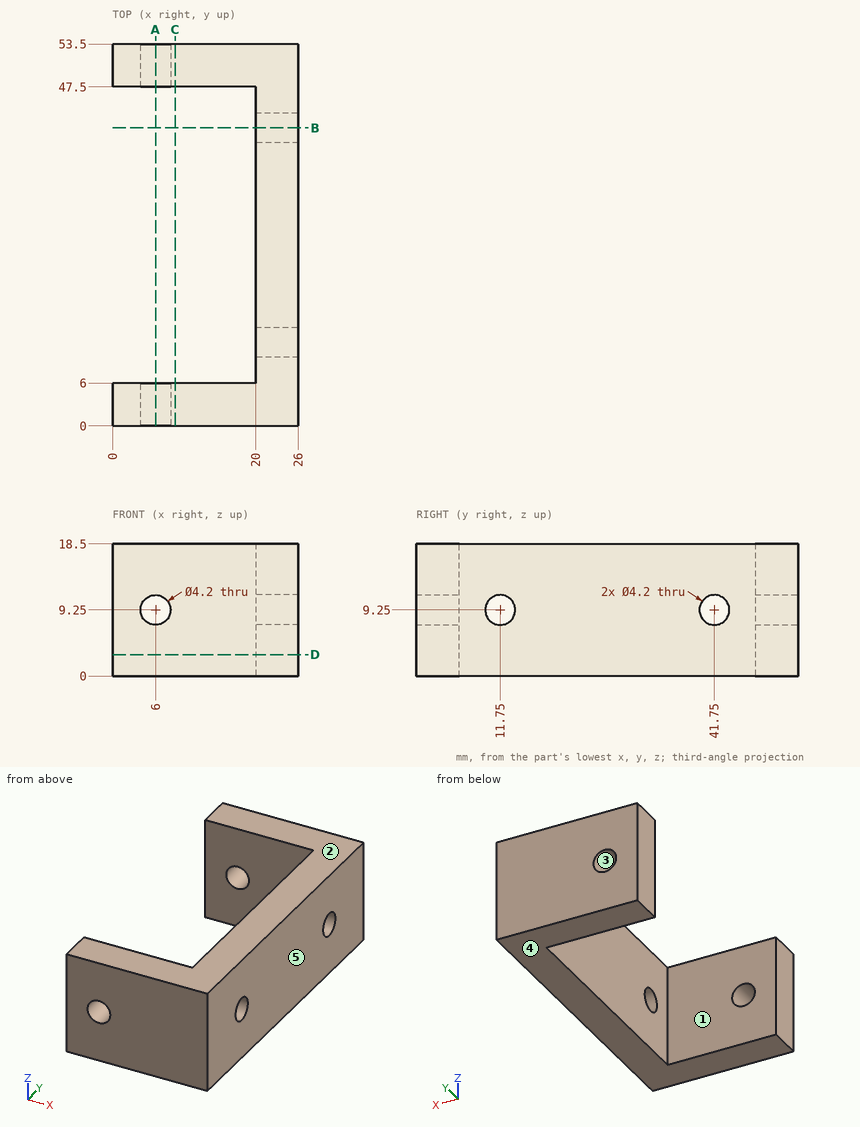
Design review of the part shown in the three views and the two pictorial views. Dimensions are in mm from the part's minimum x, y and z. A direction names the side the tool comes from. Round coordinates to 2 decimals unless told otherwise and drop trailing zeros. Write each loop counter-clockwise with the first axis right and the second up, starting at its lowest first coordinate (ties: lowest second). Pieces come first, ordered by that corner, then holes. Notation, with made-up numbers: (42.5, 43) -> (50.5, 43) arc R26 cw to (50.5, 78) -> close; hole circle Ø11 at (29, -20). An arc over 180 degrees is marked (long way). One line per question, with ' | ' between items. Start each with the question number.
1) Machinability: for the marked faces 1 and 2, which of the approach directions +Z, -Z, +X, -X, +Y, -Y give a long, thin tool a straight path to every point of the face, cutting with its end or side? Answer none if there is none.
2) Mouldability with a two-part tool opening along X and no side actions: class the marked faces 3, 4 and 5 as +X half, -X half, draft (parallel to the pull), parting line (faces both ways), or undercut.
3) Add section A-A (x = 6). Write out the cut boundary in (y, z).
4) Add section D-D (z = 3). Write out the cut boundary in (x, y).
5) Add section C-C (x = 8.75). Write out the cut boundary in (y, z), and give its area (3 significant figures).
6) Wall thickness on line 1 along Y through (x, z) = (10.5, 16); line 2 along Z through (x, y) = (6, 3.9); line 3 along X through (y, z) = (48.7, 9.25): over which ranges is each line inside the solid? List them lowest first.
7) For pin 1 Ø6.5 at (x, z) = (6, 9.25) entering from -Y; pin 2 Ø2.5 at (x, z) = (6, 9.25) entering from -Y; pin 3 Ø8 at (y, z) = (36, 2.5) entering from -X, all flat-tipped, find the tip position at first contact; note any pin that passes through.
8) Add section B-B (y = 41.75). Write out the cut boundary in (x, z), and give its area (3 significant figures).
Reported:
1) face 1: +Z, -Z, -X | face 2: +Z, +X, -X, +Y, -Y
2) face 3: undercut | face 4: draft | face 5: +X half
3) outline: (0, 0) -> (6, 0) -> (6, 7.15) -> (0, 7.15) -> close; (0, 11.35) -> (6, 11.35) -> (6, 18.5) -> (0, 18.5) -> close; (47.5, 0) -> (53.5, 0) -> (53.5, 7.15) -> (47.5, 7.15) -> close; (47.5, 11.35) -> (53.5, 11.35) -> (53.5, 18.5) -> (47.5, 18.5) -> close
4) outline: (0, 0) -> (26, 0) -> (26, 53.5) -> (0, 53.5) -> (0, 47.5) -> (20, 47.5) -> (20, 6) -> (0, 6) -> close
5) outline: (0, 0) -> (6, 0) -> (6, 18.5) -> (0, 18.5) -> close; (47.5, 0) -> (53.5, 0) -> (53.5, 18.5) -> (47.5, 18.5) -> close | area: 222 mm²
6) line 1: y = 0 to 6, 47.5 to 53.5 | line 2: z = 0 to 7.15, 11.35 to 18.5 | line 3: x = 0 to 3.9, 8.1 to 26
7) pin 1: stops at y = 0 | pin 2: passes through | pin 3: stops at x = 20
8) outline: (20, 0) -> (26, 0) -> (26, 7.15) -> (20, 7.15) -> close; (20, 11.35) -> (26, 11.35) -> (26, 18.5) -> (20, 18.5) -> close | area: 85.8 mm²
